from build123d import *

# Parameters (mm, degrees)
CYLINDER_R          = 2
CYLINDER_DEPTH      = 10
CYLINDER_ROLL_ANGLE = 90


with BuildPart() as part:
    # Cylinder → Cylinder (new body)
    with BuildSketch(Plane.XY):
        Circle(CYLINDER_R)
    extrude(amount=CYLINDER_DEPTH)


with BuildPart() as part_1:
    # Cylinder roll: moved
    add(part.part.rotate(Axis((0, 0, 0), (1, 0, 0)), CYLINDER_ROLL_ANGLE))


with BuildPart() as part_2:
    # Cylinder placement: moved
    add(part_1.part)


solid = part_2.part
Part model, mm, in its own coordinate system. Coordinates: 2 decimals unless noted, no trailing zeros. Write each loop counter-clockwise with the first axis right and the second up, starting at its lowest first coordinate (ties: lowest second). Pieces come first, ordered by that corner, then holes. Notation, with made-up numbers: (44, 14) - (61, 14) arc R29 cw to (61, 49) - close; hole circle Ø9 at (-25, 51). An arc over 180 degrees is marked (long way). Put each result on its own line as item: value.
1. Probe line 1 along X through (y, z) = (-1.5, -0.35); line 2 along Z through (x, y) = (-1.25, -2.25); line 3 along X through (y, z) = (-1.5, 1.6). List the from-to ranges inside material, lowest first. Write a range as [from, to].
Final values:
line 1: x = [-1.97, 1.97]
line 2: z = [-1.56, 1.56]
line 3: x = [-1.2, 1.2]
2. Flat gauge pin, fed straight in: pin 1 Ø1.5 at (y, z) = (-4, 1) entering from +X. Where does the tip first touch, or does it go through?
Final values:
pin 1: stops at x = 1.98
3. Band-saw the part on C-C (x = 0.7). Write the cut outline in (y, z), then the cut area to 3 significant figures.
Final values:
outline: (-10, -1.87) - (0, -1.87) - (0, 1.87) - (-10, 1.87) - close
area: 37.5 mm²
4. Band-saw the part on B-B (y = -1). Write the cut outline in (x, z), then the cut area to 3 significant figures.
Final values:
outline: circle Ø4 at (0, 0)
area: 12.6 mm²
5. Band-saw the part on A-A (z = 1.6). Write the cut outline in (x, y).
Final values:
outline: (-1.2, -10) - (1.2, -10) - (1.2, 0) - (-1.2, 0) - close
